Study the drawing (mm; zero at the part's minimum x, y, z) and answer. A direction names the side the tool comes from. Coordinates: 2 decimals unless noted, no trailing zeros. Loops run counter-clockwise (first coordinate to the right, second up) from the corner with the lowest first, then second, coordinate; pieces in that order, holes last. Notation, with made-up numbers: (78.25, 62) - (116.25, 62) arc R31 cw to (116.25, 94) - close; hole circle Ø3 at (14.25, 46.25). An arc over 180 degrees is marked (long way). Put each result on its own line as item: value.
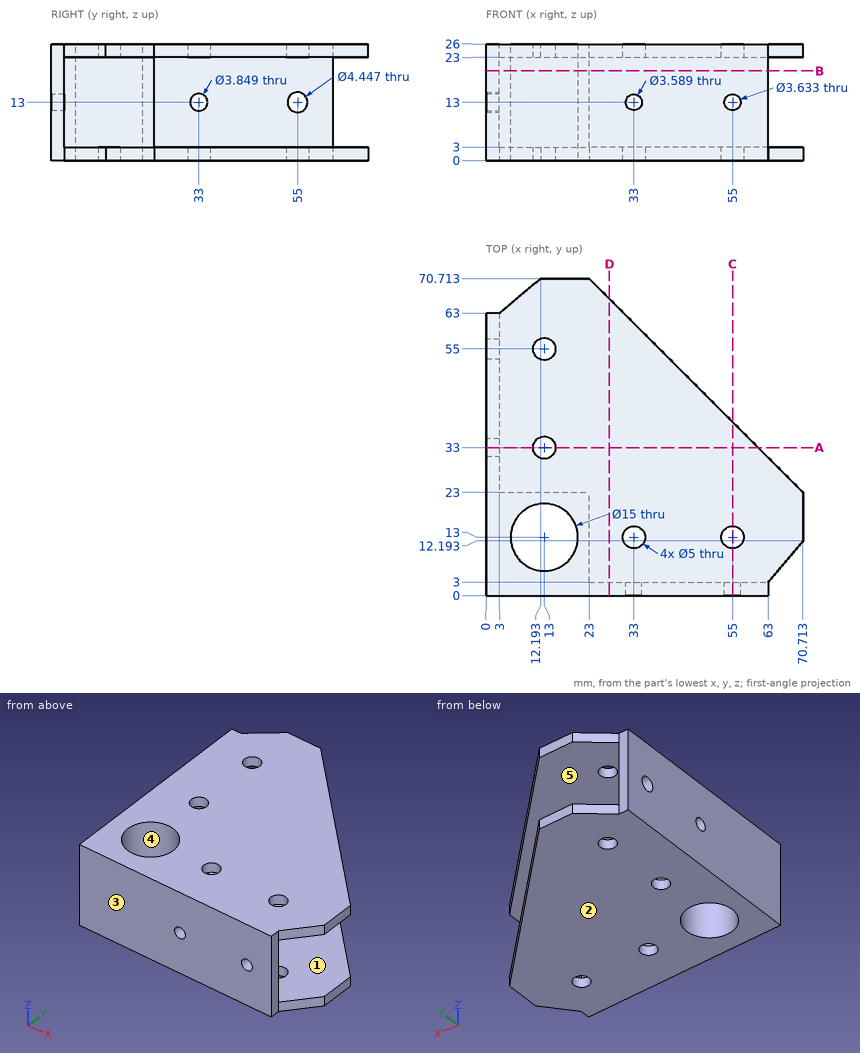
1) Each of these flat-tipped pins is pushed along its axis until it touches: pin 1 (7 mm diameter, centred on y = 55, z = 13, fed in from +X); pin 2 (13.5 mm diameter, centred on x = 13, y = 13, fed in from -Z); pin 3 (4 mm diameter, centred on x = 11, z = 7, fed in from +Y); pin 4 (4 mm diameter, centred on x = 33, z = 13, fed in from +Y). Where does it stop, or does it pass through?
Found:
pin 1: stops at x = 3
pin 2: passes through
pin 3: stops at y = 23
pin 4: stops at y = 3
2) The part is cut by section B-B (z = 20). Give the vertices of the cut face in (x, y).
Found:
outline: (0, 0) - (63, 0) - (63, 3) - (23, 3) - (23, 23) - (3, 23) - (3, 63) - (0, 63) - close; hole circle Ø15 at (13, 13)
3) Straight lines are drawn through the part: L1, parallel to X at y = 0.75, z = 13 (1 decimal); L2, parallel to Z at x = 29, y = 58; L3, parallel to Z at x = 2, y = 55. For each, find the intervals that lie inside material, in ascending order. Write a range as [from, to].
Found:
L1: x = [0, 31.2], [34.8, 53.2], [56.8, 63]
L2: z = [0, 3], [23, 26]
L3: z = [0, 10.78], [15.22, 26]
4) The part is cut by section A-A (y = 33). Give the vertices of the cut face in (x, z) (1 decimal).
Found:
outline: (0, 0) - (10.5, 0) - (10.5, 3) - (3, 3) - (3, 11.1) - (0, 11.1) - close; (0, 14.9) - (3, 14.9) - (3, 23) - (10.5, 23) - (10.5, 26) - (0, 26) - close; (15.5, 0) - (60.7, 0) - (60.7, 3) - (15.5, 3) - close; (15.5, 23) - (60.7, 23) - (60.7, 26) - (15.5, 26) - close
5) The part is cut by section D-D (x = 27.5). Give the vertices of the cut face in (y, z).
Found:
outline: (0, 0) - (66.21, 0) - (66.21, 3) - (3, 3) - (3, 23) - (66.21, 23) - (66.21, 26) - (0, 26) - close
6) The part is cut by section C-C (x = 55). Give the vertices of the cut face in (y, z).
Found:
outline: (0, 0) - (10.5, 0) - (10.5, 3) - (3, 3) - (3, 11.18) - (0, 11.18) - close; (0, 14.82) - (3, 14.82) - (3, 23) - (10.5, 23) - (10.5, 26) - (0, 26) - close; (15.5, 0) - (38.71, 0) - (38.71, 3) - (15.5, 3) - close; (15.5, 23) - (38.71, 23) - (38.71, 26) - (15.5, 26) - close
7) For the marked faces 1 and 2, determine the directions among +Z, -Z, +X, -X, +Y, -Y from which every point of the face is accessible in a straight line to the end or side of a thin tool.
Found:
face 1: +X, +Y
face 2: -Z, +X, -X, +Y, -Y
8) For a pull along Y with two mould halves and no side action, classify the marked faces 3, 4 and 5 as pulls with the +Y half, pulls with the -Y half, needs draft (parallel to the pull), parting line crosses it, or undercut.
Found:
face 3: pulls with the -Y half
face 4: undercut
face 5: needs draft
